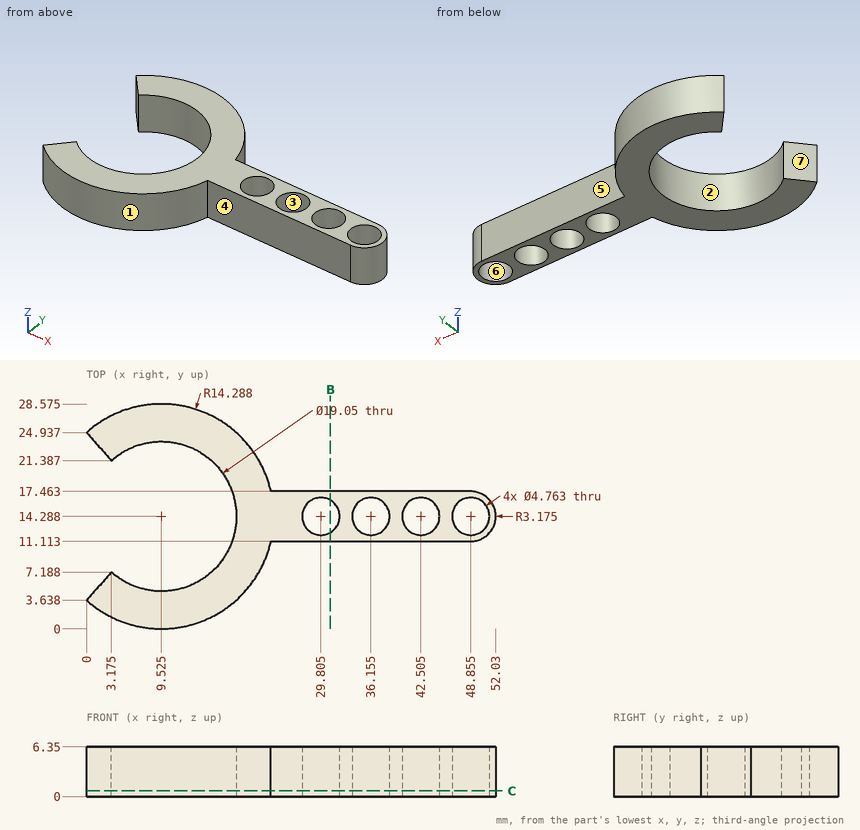
Verification items for this drawing (mm, ordinates from the low corner). A direction names the side the tool comes from. Give positions to 0.01 mm unless a question says otherwise; leave off trailing zeros. Loops run counter-clockwise (first coordinate to the right, second up) from the corner with the lowest first, then second, coordinate; pieces in that order, holes last. Notation, with made-up numbers: M 44.25,9.5 L 92.25,9.5 A17 ccw 92.25,39.5 Z; hole C -35.75,85.5 d5. An arc over 180 degrees is marked long. Write each question's results on one line, items separated by ' | '.
1) Section check C-C, the plane z = 0.75. Count the separate pieces of the cut face and the enclosed holes in it, plus the area to 3 significant figures.
Answers follow:
separate pieces: 1 | enclosed holes: 4 | area: 365 mm2
2) Section check B-B, the plane x = 31. Record the boundary of the cut face in (y, z).
Answers follow:
outline: M 11.11,0 L 12.23,0 L 12.23,6.35 L 11.11,6.35 Z; M 16.35,0 L 17.46,0 L 17.46,6.35 L 16.35,6.35 Z
3) Tool access check on the marked faces 5, 6 and 7. Record the directions out of +Z, -Z, +X, -X, +Y, -Y that give a thin tool (end or side, any length) a straight path to the whole face; none if there is none.
Answers follow:
face 5: +Z, -Z, +X, +Y | face 6: +Z, -Z | face 7: +Z, -Z, -X
4) Gauge pin test, flat ends, axial feed: pin 1 (2 mm diameter, centred on y = 11.5, z = 5, fed in from +X); pin 2 (4.5 mm diameter, centred on x = 29.81, y = 14.29, fed in from -Z); pin 3 (2 mm diameter, centred on y = 8, z = 5, fed in from -X) (1 decimal). Record the tip position at first contact, or that the pin passes through.
Answers follow:
pin 1: x = 51.48 | pin 2: through | pin 3: x = 3
5) Release check for a two-part mould opening along X. For the marked faces 1, 2, 3 and 4 record: +X half, -X half, draft (parallel to the pull), parting line (faces both ways), or undercut.
Answers follow:
face 1: parting line | face 2: undercut | face 3: undercut | face 4: draft
6) Thickness scan on line 1 (X direction, y = 14.5, z = 6); line 2 (Y direction, x = 42.5, z = 1.5); line 3 (Y direction, x = 4.5, z = 5.75) (1 decimal). Record the ranges inside material, lowest first.
Answers follow:
line 1: 19.05 to 27.43, 32.18 to 33.78, 38.53 to 40.13, 44.88 to 46.48, 51.23 to 52.02 | line 2: 11.11 to 11.91, 16.67 to 17.46 | line 3: 0.9 to 6.2, 22.4 to 27.7
